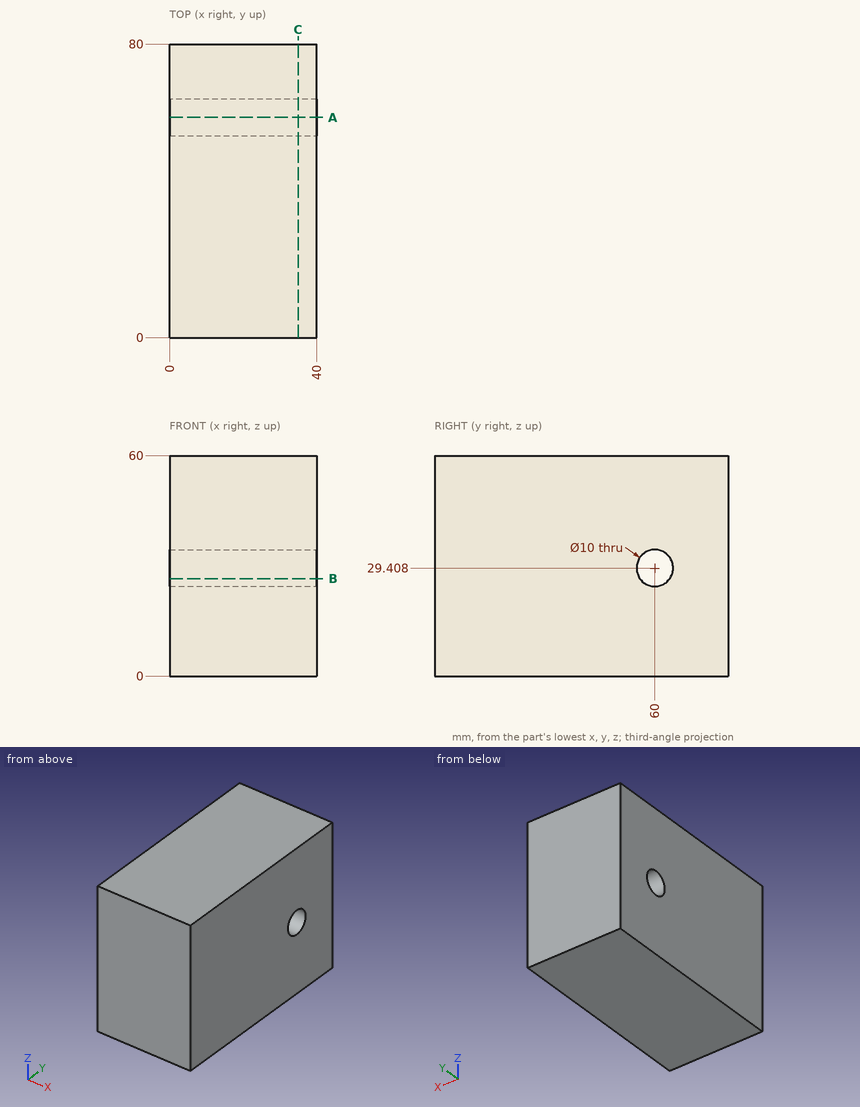
Geometry check sheet. Reference: drawing and pictorial views, mm from the part's lowest x, y, z. Give positions to 0.01 mm unless a question says otherwise; leave off trailing zeros. Order: outer loops, then holes, each group sorted by start corner. A loop starts at its lowest first (then second) coordinate and runs counter-clockwise, first axis right, second up. Notation, with made-up numbers: M -34,-34.75 L 1,-34.75 A23 ccw 1,-2.75 Z; hole C -21,37.25 d6. An arc over 180 degrees is marked long. Answer in a Markdown table with one row per item. Add a question column.
Q1. Sectioned sample at C-C, the plane x = 35. Record the boundary of the cut face in (y, z).
Q2. Sectioned sample at B-B, the plane z = 26.5. Record the boundary of the cut face in (x, y), and give its area (3 significant figures).
Q3. Thickness scan on L1, parallel to Z at x = 16, y = 60; L2, parallel to Y at x = 30, z = 32.5; L3, parallel to Y at x = 13.5, z = 28.5. Record the ranges inside material, lowest first.
Q4. Sectioned sample at A-A, the plane y = 60. Record the boundary of the cut face in (x, z), and give its area (3 significant figures).
Verdict:
| question | item | result |
|---|---|---|
| 1 | outline | M 0,0 L 80,0 L 80,60 L 0,60 Z; hole C 60,29.41 d10 |
| 2 | outline | M 0,0 L 40,0 L 40,55.93 L 0,55.93 Z; M 0,64.07 L 40,64.07 L 40,80 L 0,80 Z |
| 2 | area | 2,870 mm² |
| 3 | L1 | 0 to 24.41, 34.41 to 60 |
| 3 | L2 | 0 to 56.07, 63.93 to 80 |
| 3 | L3 | 0 to 55.08, 64.92 to 80 |
| 4 | outline | M 0,0 L 40,0 L 40,24.41 L 0,24.41 Z; M 0,34.41 L 40,34.41 L 40,60 L 0,60 Z |
| 4 | area | 2,000 mm² |
